```python
from build123d import *

# Parameters (mm, degrees)
F0_R           = 1.5
F1_DEPTH       = 18.5
F2_D           = 2.5
F3_D           = 2.5
F3_CSINK_D     = 6.72
F3_CSINK_ANGLE = 90
F4_R           = 5
F5_R           = 0.5


with BuildPart() as f1:
    # F0 (on Top) → F1 (new body)
    with BuildSketch(Plane.XY):
        with BuildLine():
            Line((-14.5, -4), (8, -4))
            ThreePointArc((8, -4), (12, 0), (8, 4))
            Line((8, 4), (-11.5, 4))
            Line((-11.5, 4), (-11.5, 16))
            Line((-11.5, 16), (-14.5, 16))
            Line((-14.5, 16), (-14.5, -4))
        make_face()
        with Locations((-8, 0)):
            Circle(F0_R, mode=Mode.SUBTRACT)
        Circle(F0_R, mode=Mode.SUBTRACT)
        with Locations((8, 0)):
            Circle(F0_R, mode=Mode.SUBTRACT)
        Circle(F0_R)
        with Locations((8, 0)):
            Circle(F0_R)
        with Locations((-8, 0)):
            Circle(F0_R)
    extrude(amount=F1_DEPTH)

    # F2 (through all)
    with Locations(Plane(origin=(0, 0, 0), x_dir=(1, 0, 0), z_dir=(0, 0, -1))):
        with Locations((8, 0), (0, 0)):
            Hole(F2_D / 2)

    # F3 (through all)
    with Locations(Plane(origin=(0, 0, 0), x_dir=(1, 0, 0), z_dir=(0, 0, -1))):
        with Locations((-8, 0)):
            CounterSinkHole(F3_D / 2, F3_CSINK_D / 2, counter_sink_angle=F3_CSINK_ANGLE)

    # F4
    f4_edges = [f1.edges().sort_by_distance(p)[0] for p in [
        (-11.5, 4, 9.25),
        (-13, 16, 18.5),
    ]]
    fillet(f4_edges, radius=F4_R)

    # F5
    f5_edges = [f1.edges().sort_by_distance(p)[0] for p in [
        (-3.25, -4, 18.5),
        (-14.5, 3.5, 18.5),
        (-14.5, 14.535534, 17.035534),
        (-14.5, -4, 9.25),
    ]]
    fillet(f5_edges, radius=F5_R)


solid = f1.part
```
Geometry check sheet. Reference: the model listing, model coordinates, mm. A direction names the side the tool comes from. Give positions to 0.01 mm unless a question says otherwise; leave off trailing zeros. Loops run counter-clockwise (first coordinate to the right, second up) from the corner with the lowest first, then second, coordinate; pieces in that order, holes last. Notation, with made-up numbers: M -34.5,58 L 22.5,58 A10 ccw 22.5,63 Z; hole C 66.25,-24.5 d10. An arc over 180 degrees is marked long. Answer as CSV lines item,"result".
Item 1: Access from +Z, -Z, +X, -X, +Y, -Y to the whole of each face (thin tool, end or side, straight path). Record for faces 4 (the flat face through (1, 4, 9)), 5 (the cylindrical face through (12, 0, 9)).
Values:
face 4,"+Z, -Z, +X, +Y"
face 5,"+Z, -Z, +X"
Item 2: Cross-section at B-B on x = 0. Record the cut outline in (y, z).
Values:
outline,"M -4,0 L -1.25,0 L -1.25,18.5 L -3.5,18.5 A0.5 ccw -4,18 Z; M 1.25,0 L 4,0 L 4,18 A0.5 ccw 3.5,18.5 L 1.25,18.5 Z"
Item 3: Cross-section at D-D on y = 9.5. Record the cut outline in (x, z), and give its area (3 significant figures).
Values:
outline,"M -14.5,0 L -11.5,0 L -11.5,18 A0.5 ccw -12,18.5 L -14,18.5 A0.5 ccw -14.5,18 Z"
area,"55.4 mm²"
Item 4: Cross-section at A-A on y = 0. Record the cut outline in (x, z), and give its area (3 significant figures).
Values:
outline,"M -14.5,0 L -11.36,0 L -9.25,2.11 L -9.25,18.5 L -14,18.5 A0.5 ccw -14.5,18 Z; M -6.75,2.11 L -4.64,0 L -1.25,0 L -1.25,18.5 L -6.75,18.5 Z; M 1.25,0 L 6.75,0 L 6.75,18.5 L 1.25,18.5 Z; M 9.25,0 L 12,0 L 12,18 A0.5 ccw 11.5,18.5 L 9.25,18.5 Z"
area,"347 mm²"
Item 5: Material ranges on line 1 (Y direction, x = 0, z = 10.5); line 2 (Y direction, x = -6, z = 2); line 3 (X direction, y = 10, z = 8.5), recorded low to high.
Values:
line 1,"y = -4 to -1.25, 1.25 to 4"
line 2,"y = -4 to 4"
line 3,"x = -14.5 to -11.5"
Item 6: Release check for a two-part mould opening along Y. For faces 1 (the flat face through (-14.5, 6, 9)), 2 (the cylindrical face through (-6.75, -0.05, 10.42)), 3 (the flat face through (-13, 16, 7)) record: pulls with the +Y half, pulls with the -Y half, needs draft (parallel to the pull), parting line crosses it, or undercut.
Values:
face 1,"needs draft"
face 2,"undercut"
face 3,"pulls with the +Y half"
Item 7: Depth check by flat-ended pin: P1, Ø4, axis at y = 8, z = 16, coming from the +X side; P2, Ø2, axis at y = 11, z = 11.5, coming from the +X side; P3, Ø2, axis at x = 0, y = 0, coming from the +Z side. Enter the tip coordinate at first touch or a pass-through.
Values:
P1,"stops at x = -10.5"
P2,"stops at x = -11.5"
P3,"passes through"
Item 8: Cross-section at C-C on z = 11.5. Record the cut outline in (x, y).
Values:
outline,"M -14.5,-3.5 A0.5 ccw -14,-4 L 8,-4 A4 ccw 8,4 L -6.5,4 A5 cw -11.5,9 L -11.5,15.5 A0.5 ccw -12,16 L -14,16 A0.5 ccw -14.5,15.5 Z; hole C -8,0 d2.5; hole C 0,0 d2.5; hole C 8,0 d2.5"
